Read the model definition and answer for the solid it produces. Units are mm, in the model's axes. A direction names the side the tool comes from. Coordinates: 2 decimals unless noted, no trailing zeros. Loops run counter-clockwise (first coordinate to the right, second up) from the corner with the lowest first, then second, coordinate; pieces in that order, holes last.
Autodesk Inventor part; units mm, degrees
ref_plane "YZ Plane" through (0, 0, 0) normal (1, 0, 0) x (0, 1, 0)
ref_plane "XZ Plane" through (0, 0, 0) normal (0, 1, 0) x (-1, 0, 0)
ref_plane "XY Plane" through (0, 0, 0) normal (0, 0, 1) x (1, 0, 0)
sketch "Sketch1" plane through (0, 0, 0) normal (0, 1, 0) x (-1, 0, 0)
  line L0 (21, -18) -> (-21, -18)
  line L1 (-21, -18) -> (-21, 18)
  line L2 (-21, 18) -> (21, 18)
  line L3 (21, 18) -> (21, -18)
  line L4 (0, -18) -> (0, 18) construction
  line L5 (21, 0) -> (-21, 0) construction
  point P0 (0, 0)
  point P1 (0, 0)
  dimension "d0" = 42
  dimension "d1" = 36
extrude "Extrusion1" add sketch "Sketch1" along normal blind 28
sketch "Sketch2" plane through (-21, 0, 18) normal (0, 0, 1) x (1, 0, 0)
  line L0 (42, 28) -> (0, 28)
  line L1 (21, 28) -> (21, 0) construction
  line L2 (0, 0) -> (0, 28)
  line L3 (0, 13) -> (42, 13) construction
  circle A0 centre (21, 13) radius 11
  dimension "d4" = 15
  dimension "d5" = 22
extrude "Extrusion2" cut sketch "Sketch2" against normal up to next
sketch "Sketch3" plane through (0, 28, 0) normal (0, 1, 0) x (1, 0, 0)
  line L0 (-15.25, 13) -> (15.25, 13) construction
  line L1 (15.25, 13) -> (15.25, -13) construction
  line L2 (15.25, -13) -> (-15.25, -13) construction
  line L3 (-15.25, -13) -> (-15.25, 13) construction
  line L4 (0, 13) -> (0, -13) construction
  line L5 (-15.25, 0) -> (15.25, 0) construction
  circle A0 centre (-15.25, 13) radius 2.15
  circle A1 centre (-15.25, -13) radius 2.15
  circle A2 centre (15.25, 13) radius 2.15
  circle A3 centre (15.25, -13) radius 2.15
  point P0 (0, 0)
  point P1 (0, 0)
  dimension "d8" = 26
  dimension "d9" = 30.5
  dimension "d10" = 4.3
  dimension "d11" = 4.3
  dimension "d12" = 4.3
  dimension "d13" = 4.3
extrude "Extrusion3" cut sketch "Sketch3" against normal up to next
sketch "Sketch4" plane through (0, 28, 0) normal (0, 1, 0) x (1, 0, 0)
  circle A0 centre (15.25, -13) radius 2.15
  circle A1 centre (15.25, -13) radius 2.5
  circle A2 centre (-15.25, -13) radius 2.15
  circle A3 centre (-15.25, -13) radius 2.5
  circle A4 centre (15.25, 13) radius 2.15
  circle A5 centre (15.25, 13) radius 2.5
  circle A6 centre (-15.25, 13) radius 2.15
  circle A7 centre (-15.25, 13) radius 2.5
  point P0 (0, 0)
  dimension "d16" = 5
  dimension "d17" = 5
  dimension "d18" = 5
  dimension "d19" = 5
extrude "Extrusion5" cut sketch "Sketch4" against normal blind 12 contours A1 | A3 | A4 | A5 | A7
sketch "Sketch5" plane through (-21, 0, 18) normal (0, 0, 1) x (1, 0, 0)
  line L0 (0, 28) -> (42, 28) construction
  line L1 (21, 28) -> (21, 0) construction
  line L2 (42, 0) -> (0, 0) construction
  line L3 (0, 28) -> (0, 20)
  line L4 (0, 0) -> (0, 28)
  line L5 (21, 0) -> (14.5, 0)
  line L6 (10.5, 4) -> (14.5, 0)
  line L7 (0, 20) -> (1, 19)
  line L8 (1, 19) -> (1, 4)
  line L9 (1, 4) -> (10.5, 4)
  line L10 (0, 20) -> (0, 0)
  line L11 (14.5, 0) -> (0, 0)
  line L12 (0, 0) -> (42, 0) construction
  line L13 (42, 0) -> (42, 28)
  line L14 (31.5, 4) -> (27.5, 0)
  line L15 (42, 20) -> (41, 19)
  line L16 (41, 19) -> (41, 4)
  line L17 (41, 4) -> (31.5, 4)
  line L18 (27.5, 0) -> (42, 0)
  dimension "d27" = 8
  dimension "d28" = 9
  dimension "d29" = 135
  dimension "d35" = 9.5
  dimension "d43" = 135
  dimension "d44" = 24
extrude "Extrusion7" cut sketch "Sketch5" against normal up to next
sketch "Sketch6" plane through (0, 28, 0) normal (0, 1, 0) x (1, 0, 0)
  line L0 (6.5, -18) -> (10.5, -18)
  circle A0 centre (15.25, -13) radius 2.5 construction
  line L1 (15.25, -13) -> (15.25, -18) construction
  line L2 (-21, -18) -> (21, -18) construction
  line L3 (21, 18) -> (-21, 18)
  line L4 (9.5, 18) -> (-9.5, 18)
  line L5 (-9.5, 18) -> (-9.5, -18)
  line L6 (-9.5, -18) -> (9.5, -18)
  line L7 (9.5, -18) -> (9.5, 18)
  line L8 (0, -18) -> (0, 18) construction
  line L9 (0, 18) -> (0, -18) construction
  point P0 (0, 0)
  dimension "d36" = 5.75
extrude "Extrusion8" cut sketch "Sketch6" against normal blind 1
sketch "Sketch7" plane through (6.5, 0, -18) normal (0, 0, -1) x (-1, 0, 0)
  line L0 (16, 27) -> (-3, 27)
  line L1 (-3, 28) -> (-14.5, 28)
  line L2 (-3, 27) -> (-3, 28)
  line L3 (-3, 27) -> (-2, 27)
  line L4 (-2, 27) -> (-3, 28)
  line L5 (-3, 27) -> (-3, 28) construction
  line L6 (27.5, 28) -> (16, 28) construction
  line L7 (-3, 28) -> (16, 28) construction
  line L8 (6.5, 28) -> (6.5, 27) construction
  line L9 (-3, 27) -> (16, 27)
  line L10 (16, 27) -> (16, 28)
  line L11 (15, 27) -> (16, 28)
  line L12 (15, 27) -> (16, 27) construction
  point P0 (6.5, 0)
  dimension "d39" = 1
extrude "Extrusion9" add sketch "Sketch7" against normal blind 36
thread "Thread1"
thread "Thread2"
thread "Thread3"
thread "Thread4"
properties part number "SC12UU"
Q1. Straight lines are drawn through the part: probe 1 along Z at (x, y) = (15.25, 9.75); probe 2 along Z at (x, y) = (15.25, 22.25); probe 3 along Y at (x, z) = (0, 5.5). For each, find the intervals that lie inside material, in ascending order.
Findings below:
probe 1: z = -18 to -15.15, -10.85 to 10.85, 15.15 to 18
probe 2: z = -18 to -15.5, -10.5 to 10.5, 15.5 to 18
probe 3: y = 0 to 2, 24 to 27
Q2. A cutting plane is placed at A-A (y = 13). Give the vertices of the cut face in (x, z), then the cut area to 3 significant figures.
Findings below:
outline: (-20, -18) - (-11, -18) - (-11, 18) - (-20, 18) - close; (11, -18) - (20, -18) - (20, 18) - (11, 18) - close; hole circle Ø4.3 at (-15.25, -13); hole circle Ø4.3 at (-15.25, 13); hole circle Ø4.3 at (15.25, -13); hole circle Ø4.3 at (15.25, 13)
area: 590 mm2
Q3. Determine the mould class of faces 4 (the face through (-8.5, 2, 0.3)), 5 (the face through (13.266, 22.084, -11.479)) for opening direction Z: +Z half, -Z half, draft (parallel to the pull), parting line (faces both ways), or undercut.
Findings below:
face 4: draft
face 5: undercut
Q4. A cutting plane is placed at B-B (x = -15.25). Give the vertices of the cut face in (y, z), then the cut area to 3 significant figures.
Findings below:
outline: (4, -18) - (28, -18) - (28, -15.5) - (16, -15.5) - (16, -15.15) - (4, -15.15) - close; (4, -10.85) - (16, -10.85) - (16, -10.5) - (28, -10.5) - (28, 10.5) - (16, 10.5) - (16, 10.85) - (4, 10.85) - close; (4, 15.15) - (16, 15.15) - (16, 15.5) - (28, 15.5) - (28, 18) - (4, 18) - close
area: 641 mm2
Q5. Which of the six approach directions +Z, -Z, +X, -X, +Y, -Y give full straight-line access (tool end or side, diameter ignored) to faces 1 (the face through (-20, 12, 0)), 2 (the face through (-9, 27.5, -0.3)), 3 (the face through (-17.234, 22.084, 14.521))?
Findings below:
face 1: +Z, -Z, -X, -Y
face 2: +Z, -Z, +Y
face 3: +Y
Q6. Flat-ended cylindrical pins translate along their axes: pin 1 Ø12 at (y, z) = (9.5, -7) entering from +X; pin 2 Ø4.5 at (x, z) = (-15.25, -13) entering from -Y; pin 3 Ø7 at (x, z) = (-15.25, 13) entering from +Y; pin 4 Ø6 at (y, z) = (11.5, -3.5) entering from -X. Find the tip coordinate at first contact, or state that the pin passes through.
Findings below:
pin 1: stops at x = 20
pin 2: stops at y = 4
pin 3: stops at y = 28
pin 4: stops at x = -20
Q7. A cutting plane is placed at D-D (z = -6.5). Give the vertices of the cut face in (x, y), then the cut area to 3 significant figures.
Findings below:
outline: (-21, 20) - (-20, 19) - (-20, 4) - (-10.5, 4) - (-6.5, 0) - (6.5, 0) - (10.5, 4) - (20, 4) - (20, 19) - (21, 20) - (21, 28) - (9.5, 28) - (8.5, 27) - (-8.5, 27) - (-9.5, 28) - (-21, 28) - close; hole circle Ø22 at (0, 13)
area: 647 mm2
Q8. A cutting plane is placed at C-C (z = 13). Count the separate pieces of the cut face and the enclosed holes in it, then the cut area to 3 significant figures.
Findings below:
separate pieces: 3
enclosed holes: 1
area: 424 mm2
